Input: part model. Units: mm. Frame: model coordinates. A direction names the side the tool comes from. Round coordinates to 2 decimals unless told otherwise and drop trailing zeros. Write each loop counter-clockwise with the first axis right and the second up, starting at its lowest first coordinate (ties: lowest second). Pieces come first, ordered by that corner, then holes. Notation, with made-up numbers: (20.5, 87) -> (47.5, 87) arc R23 ccw to (47.5, 122) -> close; hole circle Ø5 at (-3.75, 17.5). An arc over 180 degrees is marked (long way). Write item = value, one per line.
```python
from build123d import *

# Parameters (mm, degrees)
F1_DEPTH = 25.4


with BuildPart() as f1:
    # F0 (on Top) → F1 (new body)
    with BuildSketch(Plane.XY):
        Polygon((-53.5242615514, -0.6677641515), (-27.7371538567, 46.6872522981), (-80.864693046, 46.6872522981), align=None)
        Polygon((26.1838300567, 46.6872522981), (-2.3295022303, 93.3454419237), (-27.7371538567, 46.6872522981), align=None)
        Polygon((80.864693046, 46.6872522981), (26.1838300567, 46.6872522981), (54.3009234514, 0.6774537196), align=None)
        Polygon((82.0042751486, -44.6553128522), (54.3009234514, 0.6774537196), (27.3404314946, -46.0194881465), align=None)
        Polygon((-26.5637695946, -47.3647060176), (-53.5242615514, -0.6677641515), (-79.6747729182, -48.6901290715), align=None)
        Polygon((0, -93.3745045961), (27.3404314946, -46.0194881465), (-26.5637695946, -47.3647060176), align=None)
        Polygon((54.3009234514, 0.6774537196), (26.1838300567, 46.6872522981), (-27.7371538567, 46.6872522981), (-53.5242615514, -0.6677641515), (-26.5637695946, -47.3647060176), (27.3404314946, -46.0194881465), align=None)
    extrude(amount=F1_DEPTH)


solid = f1.part
```
1) Cut plane C-C (x = -68). Return the cut outline in (y, z), and give its area (3 significant figures).
Solutions:
outline = (-48.4, 0) -> (-27.25, 0) -> (-27.25, 25.4) -> (-48.4, 25.4) -> close; (24.4, 0) -> (46.69, 0) -> (46.69, 25.4) -> (24.4, 25.4) -> close
area = 1,100 mm^2
2) Line query: L1, parallel to Y at x = -64.5, z = 2; L2, parallel to Y at x = -63, z = 15.75; L3, parallel to X at y = 69, z = 8.75. Output: solid intervals per line, ascending. Write a range as from..to.
Solutions:
L1 = -48.31..-20.82, 18.34..46.69
L2 = -48.27..-18.07, 15.74..46.69
L3 = -15.59..12.55
3) Access query for faces 5 (the face through (-54, 46.687, 13)), 6 (the face through (-1, 1, 0)), 7 (the face through (68.35, -22.31, 12.52)), 8 (the face through (-67.386, 23.341, 12.522)). Directions: +Z, -Z, +X, -X, +Y, -Y. A direction counts if a zero-diameter tool reaches every point of the face in a straight line with its end or side. Return the directions, or none.
Solutions:
face_5 = +Z, -Z, -X, +Y
face_6 = -Z, +X, -X, +Y, -Y
face_7 = +Z, -Z, +X
face_8 = +Z, -Z, -X
4) Cut plane A-A (x = 62.5). Return the cut outline in (y, z), and give its area (3 significant figures).
Solutions:
outline = (-45.14, 0) -> (-12.74, 0) -> (-12.74, 25.4) -> (-45.14, 25.4) -> close; (14.88, 0) -> (46.69, 0) -> (46.69, 25.4) -> (14.88, 25.4) -> close
area = 1,630 mm^2
5) First-contact query: P1, Ø5, axis at y = -9.5, z = 8.5, coming from the +X side; P2, Ø4, axis at y = -14.5, z = 16, coming from the -X side; P3, Ø10, axis at x = -63, z = 11.5, coming from the +Y side. Flat tips, straight axial feed; report the tip coordinate or a pass-through.
Solutions:
P1 = 62.05
P2 = -62.15
P3 = 46.69
6) Cut plane B-B (z = 14.75). Return the cut outline in (x, y).
Solutions:
outline = (-80.86, 46.69) -> (-53.52, -0.67) -> (-79.67, -48.69) -> (-26.56, -47.36) -> (0, -93.37) -> (27.34, -46.02) -> (82, -44.66) -> (54.3, 0.68) -> (80.86, 46.69) -> (26.18, 46.69) -> (-2.33, 93.35) -> (-27.74, 46.69) -> close
7) Cut plane D-D (y = -33.5). Return the cut outline in (x, z).
Solutions:
outline = (-71.4, 0) -> (75.19, 0) -> (75.19, 25.4) -> (-71.4, 25.4) -> close
8) Draft query along Y for faces 1 (the face through (67.397, 23.36, 12.522)), 2 (the face through (13.48, -70.03, 12.52)), 3 (the face through (54, 46.687, 13)), 4 (the face through (-66.416, -24.343, 12.522)). Return one class per face: +Y half, -Y half, draft (parallel to the pull), parting line (faces both ways), or undercut.
Solutions:
face_1 = undercut
face_2 = -Y half
face_3 = +Y half
face_4 = undercut
